from build123d import *

# Parameters (mm, degrees)
F0_W      = 177.8
F0_H      = 177.8
F1_DEPTH  = 76.2
F2_W      = 167.9080887029
F2_H      = 55.88
F3_DEPTH  = 176.276
F4_W      = 167.9080887029
F4_H      = 9.8836272268
F5_DEPTH  = 101.6
F6_W      = 167.2196879183
F6_H      = 10.4363727732
F7_DEPTH  = 114.3
F8_R      = 47.6089031409
F9_DEPTH  = 41.91
F10_R     = 52.5050220685
F11_DEPTH = 159.004


with BuildPart() as f1:
    # F0 (on Front) → F1 (new body)
    with BuildSketch(Plane.XZ):
        with Locations((-48.9930282295, -12.3306500904)):
            Rectangle(F0_W, F0_H)
    extrude(amount=F1_DEPTH)

    # F2 (on face) → F3 (cut)
    with BuildSketch(Plane.XY.offset(76.5693499096)):
        with Locations((-46.0179038346, -38.3763727732)):
            Rectangle(F2_W, F2_H)
    extrude(amount=-F3_DEPTH, mode=Mode.SUBTRACT)

    # F4 (on face) → F5 (join)
    with BuildSketch(Plane.XY.offset(76.5693499096)):
        with Locations((-46.0179038346, -71.2581863866)):
            Rectangle(F4_W, F4_H)
    extrude(amount=F5_DEPTH)

    # F6 (on face) → F7 (join)
    with BuildSketch(Plane.XY.offset(76.5693499096)):
        with Locations((-45.6737034423, -5.2181863866)):
            Rectangle(F6_W, F6_H)
    extrude(amount=F7_DEPTH)

    # F8 (on face) → F9 (cut)
    with BuildSketch(Plane(origin=(0, 0, 0), x_dir=(-1, 0, 0), z_dir=(0, 1, 0))):
        with Locations((38.7143976986, 134.4432979822)):
            Circle(F8_R)
    extrude(amount=-F9_DEPTH, mode=Mode.SUBTRACT)

    # F10 (on face) → F11 (cut)
    with BuildSketch(Plane.XZ.offset(76.2)):
        with Locations((-52.5096356869, 119.113817811)):
            Circle(F10_R)
    extrude(amount=-F11_DEPTH, mode=Mode.SUBTRACT)


solid = f1.part
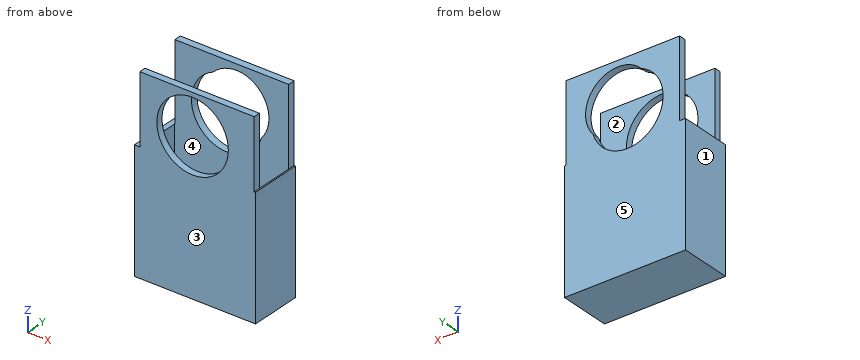
Part model, mm, in its own coordinate system. Face numbers are marked on the shaded views. A direction names the side the tool comes from. Coordinates: 2 decimals unless noted, no trailing zeros. Loops run counter-clockwise (first coordinate to the right, second up) from the corner with the lowest first, then second, coordinate; pieces in that order, holes last. Notation, with made-up numbers: (13.25, 18.5) -> (67.25, 18.5) arc R11 cw to (67.25, 27.5) -> close; hole circle Ø4 at (-21, 59.5). An arc over 180 degrees is marked (long way). Use a Markdown table: item, result. Add a question column.
Item 1: Pull direction X, two halves, no side cores. Call the marked faces 1, 2 and 3: +X half, -X half, draft (parallel to the pull), parting line (faces both ways), or undercut.
Item 2: Band-saw the part on C-C on z = 159. Write the cut outline in (x, y).
Item 3: Band-saw the part on D-D on x = 23.5. Write the cut outline in (y, z).
Item 4: Band-saw the part on B-B on y = -5. Write the cut outline in (x, z).
Item 5: Which spindle directions (+Z, -Z, +X, -X, +Y, -Y) get a long thin tool onto all of the face, cutting with end or side? Do the marked faces 4 and 5. Say none if no direction does.
Item 6: Band-saw the part on A-A on z = -54. Write the cut outline in (x, y), plus the area to 3 significant figures.
Item 7: Flat gauge pins, fed straight in: P1, Ø8.5, axis at y = -7.5, z = 110, coming from the -X side; P2, Ø5, axis at x = -66, y = -70, coming from the +Z side; P3, Ø6, axis at x = -102.5, y = -43, coming from the +Z side; P4, Ø12, axis at x = -10, z = 131, coming from the +Y side. Where does each tip first touch, or does it go through?
Item 8: Probe probe 1 along X at (y, z) = (-56.5, 0); probe 2 along Y at (x, z) = (-10, 177.5); probe 3 along Z at (x, y) = (-114, -30.5). List the from-to ranges inside material, lowest first.
Geometry says:
| question | item | result |
|---|---|---|
| 1 | face 1 | -X half |
| 1 | face 2 | undercut |
| 1 | face 3 | draft |
| 2 | outline | (-129.97, -76.2) -> (-86.65, -76.2) -> (-86.65, -66.32) -> (-129.97, -66.32) -> close; (-129.28, -10.44) -> (-86.65, -10.44) -> (-86.65, 0) -> (-129.28, 0) -> close; (-18.36, -76.2) -> (37.94, -76.2) -> (37.94, -66.32) -> (-18.36, -66.32) -> close; (2.07, -10.44) -> (37.94, -10.44) -> (37.94, 0) -> (2.07, 0) -> close |
| 3 | outline | (-76.2, -101.23) -> (0, -101.23) -> (0, 190.87) -> (-10.44, 190.87) -> (-10.44, -99.71) -> (-66.32, -99.71) -> (-66.32, 178.17) -> (-76.2, 178.17) -> close |
| 4 | outline | (-137.89, -101.23) -> (39.91, -101.23) -> (39.91, 76.57) -> (37.94, 76.57) -> (37.94, 190.87) -> (-129.28, 190.87) -> (-129.28, 76.57) -> (-137.89, 76.57) -> close; hole (-73.03, 167.44) arc R52.51 ccw (long way) to (-2.29, 103.78) arc R47.61 ccw to start |
| 5 | face 4 | +Z |
| 5 | face 5 | +Z, -Z, +X, -X, +Y |
| 6 | outline | (-137.89, -76.2) -> (39.91, -76.2) -> (39.91, 0) -> (-137.89, 0) -> close; hole (-129.97, -66.32) -> (37.94, -66.32) -> (37.94, -10.44) -> (-129.97, -10.44) -> close |
| 6 | area | 4,170 mm² |
| 7 | P1 | x = -129.28 |
| 7 | P2 | z = 178.17 |
| 7 | P3 | z = -99.71 |
| 7 | P4 | through |
| 8 | probe 1 | -137.89 to -129.97, 37.94 to 39.91 |
| 8 | probe 2 | -76.2 to -66.32, -10.44 to 0 |
| 8 | probe 3 | -101.23 to -99.71 |
